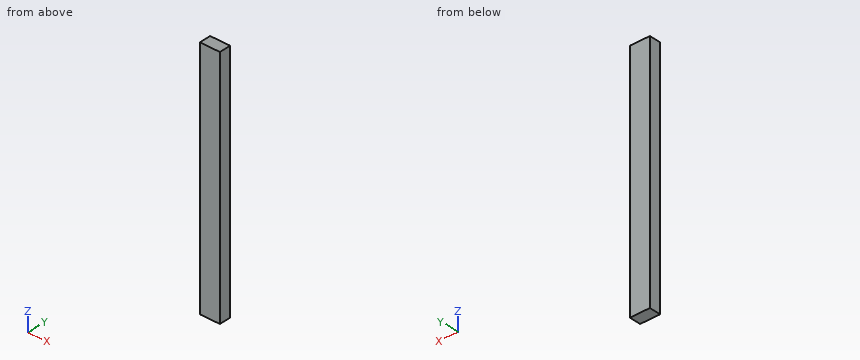
Autodesk Inventor part; units mm, degrees
ref_plane "YZ Plane" through (0, 0, 0) normal (1, 0, 0) x (0, 1, 0)
ref_plane "XZ Plane" through (0, 0, 0) normal (0, 1, 0) x (-1, 0, 0)
ref_plane "XY Plane" through (0, 0, 0) normal (0, 0, 1) x (1, 0, 0)
sketch "Sketch1" plane through (0, 0, 0) normal (0, 0, 1) x (1, 0, 0)
  line L0 (-14, -7.9) -> (14, -7.9)
  line L1 (14, -7.9) -> (14, 8.3)
  line L2 (14, 8.3) -> (-14, 8.3)
  line L3 (-14, 8.3) -> (-14, -7.9)
  line L4 (-13, 7.3) -> (13, 7.3)
  line L5 (13, 7.3) -> (13, -6.9)
  line L6 (13, -6.9) -> (-13, -6.9)
  line L7 (-13, -6.9) -> (-13, 7.3)
  dimension "d2" = 1
extrude "Extrusion1" add sketch "Sketch1" along normal blind 340
sketch "Sketch2" plane through (0, 0, 340) normal (0, 0, 1) x (1, 0, 0)
  line L0 (14, 8.3) -> (-14, 8.3) construction
  line L1 (14, -7.9) -> (14, 8.3) construction
  line L2 (-14, 8.3) -> (14, 8.3)
  line L3 (14, 8.3) -> (14, -7.9)
  line L4 (14, -7.9) -> (-14, -7.9)
  line L5 (-14, -7.9) -> (-14, 8.3)
  point P0 (0, 0)
extrude "Extrusion2" add sketch "Sketch2" against normal blind 2
sketch "Sketch3" plane through (0, 0, 0) normal (0, 0, -1) x (-1, 0, 0)
  line L0 (14, -7.9) -> (-14, -7.9) construction
  line L1 (14, -7.9) -> (-14, -7.9)
  line L2 (-14, -7.9) -> (-14, 8.3)
  line L3 (-14, 8.3) -> (14, 8.3)
  line L4 (14, 8.3) -> (14, -7.9)
  point P0 (0, 0)
extrude "Extrusion3" add sketch "Sketch3" against normal blind 2
properties part number "PL_rod_duoble"
Work out the finished part from the listing and answer in its coordinate system (mm). Round coordinates to 2 decimals unless told otherwise and drop trailing zeros. Order: outer loops, then holes, each group sorted by start corner. A loop starts at its lowest first (then second) coordinate and runs counter-clockwise, first axis right, second up.
Q1. A cutting plane is placed at B-B, the plane z = 241.5. Determine the outline of the cut face in (x, y), then the cut area to 3 significant figures.
Solution:
outline: (-14, -7.9) - (14, -7.9) - (14, 8.3) - (-14, 8.3) - close; hole (-13, -6.9) - (13, -6.9) - (13, 7.3) - (-13, 7.3) - close
area: 84.4 mm2
Q2. A cutting plane is placed at A-A, the plane x = -5.5. Determine the outline of the cut face in (y, z).
Solution:
outline: (-7.9, 0) - (8.3, 0) - (8.3, 340) - (-7.9, 340) - close; hole (-6.9, 2) - (7.3, 2) - (7.3, 338) - (-6.9, 338) - close
Q3. Find the intervals of material crossed by line 1 along X through (y, z) = (5, 151.5); line 2 along Z through (x, y) = (-10, 2.25); line 3 along Y through (x, z) = (11.5, 278.5), in increasing order.
Solution:
line 1: x = -14 to -13, 13 to 14
line 2: z = 0 to 2, 338 to 340
line 3: y = -7.9 to -6.9, 7.3 to 8.3
